Design review of the part built by this model. Coordinates are the model's own, in mm. A direction names the side the tool comes from. Give positions to 0.01 mm unless a question says otherwise; leave off trailing zeros. Order: outer loops, then holes, each group sorted by start corner. A loop starts at its lowest first (then second) coordinate and runs counter-clockwise, first axis right, second up. Notation, with made-up numbers: (-11.5, 44) -> (15.5, 44) arc R20 ccw to (15.5, 80) -> close; hole circle Ø8 at (76, 34.5). An arc over 180 degrees is marked (long way). One line per item, written item: value.
from build123d import *

# Parameters (mm, degrees)
ESTRUSIONE1_DEPTH        = 15
SMUSSO1_SIZE             = 5
SCHIZZO2_R               = 14
TAGLIO_ESTRUSIONE1_DEPTH = 59.523499554
SCHIZZO4_R               = 3
TAGLIO_ESTRUSIONE3_DEPTH = 20
SCHIZZO5_R               = 5.25
TAGLIO_ESTRUSIONE4_DEPTH = 8.5
ESTRUSIONE2_START        = -15
ESTRUSIONE2_DEPTH        = 15
SCHIZZO9_R               = 3
TAGLIO_ESTRUSIONE7_DEPTH = 10


with BuildPart() as part:
    # Schizzo1 → Estrusione1 (new body)
    with BuildSketch(Plane.XY):
        with BuildLine():
            Line((-40, 40), (0, 40))
            ThreePointArc((0, 40), (40, 0), (0, -40))
            Line((0, -40), (-40, -40))
            Line((-40, -40), (-40, 40))
        make_face()
    extrude(amount=ESTRUSIONE1_DEPTH)

    # Smusso1
    smusso1_edges = [part.edges().sort_by_distance(p)[0] for p in [
        (-40, 0, 15),
    ]]
    chamfer(smusso1_edges, length=SMUSSO1_SIZE)

    # Schizzo2 → Taglio-Estrusione1 (cut, through all)
    with BuildSketch(Plane(origin=(0, 0, 0), x_dir=(-1, 0, 0), z_dir=(0, 0, -1))):
        Circle(SCHIZZO2_R)
    extrude(amount=-TAGLIO_ESTRUSIONE1_DEPTH, mode=Mode.SUBTRACT)

    # Schizzo4 → Taglio-Estrusione3 (cut)
    with BuildSketch(Plane.XY.offset(15)):
        with Locations((-22.980970389, 22.980970389)):
            Circle(SCHIZZO4_R)
        with Locations((22.980970389, -22.980970389)):
            Circle(SCHIZZO4_R)
    extrude(amount=-TAGLIO_ESTRUSIONE3_DEPTH, mode=Mode.SUBTRACT)

    # Schizzo5 → Taglio-Estrusione4 (cut)
    with BuildSketch(Plane.XY.offset(15)):
        with Locations((-22.980970389, 22.980970389)):
            Circle(SCHIZZO5_R)
        with Locations(Location((22.980970389, -22.980970389, 0), (0, 0, 180))):
            Circle(SCHIZZO5_R)
    extrude(amount=-TAGLIO_ESTRUSIONE4_DEPTH, mode=Mode.SUBTRACT)

    # Schizzo6 → Estrusione2 (add)
    with BuildSketch(Plane.XY.offset(15).offset(ESTRUSIONE2_START)):
        with BuildLine():
            Line((11.73594132, 38.239608802), (202.93398533, -20.4400978))
            ThreePointArc((202.93398533, -20.4400978), (209.889363529, -31.483404529), (200, -40))
            Line((200, -40), (0, -40))
            ThreePointArc((0, -40), (39.557454115, -5.933618117), (11.73594132, 38.239608802))
        make_face()
    extrude(amount=ESTRUSIONE2_DEPTH)

    # Schizzo9 → Taglio-Estrusione7 (cut)
    with BuildSketch(Plane(origin=(0, 0, 0), x_dir=(-1, 0, 0), z_dir=(0, 0, -1))):
        with Locations((-57, -8.648405099)):
            Circle(SCHIZZO9_R)
        with Locations((-138.285904257, -33.5)):
            Circle(SCHIZZO9_R)
    extrude(amount=-TAGLIO_ESTRUSIONE7_DEPTH, mode=Mode.SUBTRACT)


solid = part.part
Item 1: To check wall thickness, follow line 1 along X through (y, z) = (-29.5, 9.75); line 2 along Y through (x, z) = (-2, 10); line 3 along Y through (x, z) = (137, 2.5). State the ranges of each line that lie inside material, in increasing order. Write a range as from..to.
Returned:
line 1: -40..209.99
line 2: -40..-13.86, 13.86..40
line 3: -40..-36.21, -30.79..-0.2
Item 2: Add section C-C on z = 3.5. Give the boundary of the cut face in (x, y).
Returned:
outline: (-40, -40) -> (200, -40) arc R10 ccw to (202.93, -20.44) -> (11.74, 38.24) arc R40 ccw to (0, 40) -> (-40, 40) -> close; hole circle Ø6 at (-22.98, 22.98); hole circle Ø28 at (0, 0); hole circle Ø6 at (22.98, -22.98); hole circle Ø6 at (57, -8.65); hole circle Ø6 at (138.29, -33.5)
Item 3: Machinability: for faces 1 (the cylindrical face through (-25.98, 23.11, 3.3)), 2 (the flat face through (20.7, -20.7, 6.5)), 3 (the flat face through (138, -33, 10)), which of the approach directions +Z, -Z, +X, -X, +Y, -Y give a long, thin tool a straight path to every point of the face, cutting with its end or side? Answer none if there is none.
Returned:
face 1: +Z, -Z
face 2: +Z
face 3: -Z
Item 4: Add section B-B on y = -33.5. Give the boundary of the cut face in (x, z), plus the area to 3 significant figures.
Returned:
outline: (-40, 0) -> (135.29, 0) -> (135.29, 10) -> (141.29, 10) -> (141.29, 0) -> (209.37, 0) -> (209.37, 15) -> (-35, 15) -> (-40, 10) -> close
area: 3,670 mm²
Item 5: Add section D-D on x = 57. Give the boundary of the cut face in (y, z).
Returned:
outline: (-40, 0) -> (-11.65, 0) -> (-11.65, 10) -> (-5.65, 10) -> (-5.65, 0) -> (24.35, 0) -> (24.35, 15) -> (-40, 15) -> close
Item 6: Add section A-A on y = 9. Give the boundary of the cut face in (x, z), plus the area to 3 significant figures.
Returned:
outline: (-40, 0) -> (-10.72, 0) -> (-10.72, 15) -> (-35, 15) -> (-40, 10) -> close; (10.72, 0) -> (107.01, 0) -> (107.01, 15) -> (10.72, 15) -> close
area: 1,870 mm²
Item 7: Clearance check with flat-ended pins moving along their axes: P1, Ø6.5, axis at x = 22.98, y = -22.98, coming from the +Z side; P2, Ø1.8, axis at x = 58, y = -8, coming from the -Z side; P3, Ø3, axis at x = -22, y = 24, coming from the +Z side. State where each tip first meets the part, or that it passes through.
Returned:
P1: z = 6.5
P2: z = 10
P3: through
Item 8: Draft analysis for pull direction Y (two halves, no side actions). For faces 4 (the cylindrical face through (209.917, -31.286, 7.395)), 5 (the cylindrical face through (59.997, -8.517, 4.93)), 6 (the flat face through (-37, -1, 13)), state which applies: pulls with the +Y half, pulls with the -Y half, needs draft (parallel to the pull), parting line crosses it, or undercut.
Returned:
face 4: parting line crosses it
face 5: undercut
face 6: needs draft
